Read the model definition and answer for the solid it produces. Units are mm, in the model's axes. Give positions to 0.01 mm unless a question says otherwise; leave off trailing zeros. Order: outer loops, then holes, each group sorted by start corner. A loop starts at its lowest first (then second) coordinate and runs counter-clockwise, first axis right, second up. Notation, with made-up numbers: (-18.5, -2.75) - (38.5, -2.75) arc R14 cw to (38.5, 5.25) - close; hole circle Ø9 at (-36.75, 85.5). An arc over 180 degrees is marked (long way). Write item = value, one per line.
```python
from build123d import *

# Parameters (mm, degrees)
F0_W     = 1250
F0_H     = 450
F1_DEPTH = 19
F3_DEPTH = 19
F5_DEPTH = 19
F7_D     = 10
F7_DEPTH = 13
F7_TIP   = 3.0043030951


with BuildPart() as f1:
    # F0 (on Top) → F1 (new body)
    with BuildSketch(Plane.XY):
        Rectangle(F0_W, F0_H)
    extrude(amount=F1_DEPTH)

    # F2 (on face) → F3 (cut, through all)
    with BuildSketch(Plane.XY.offset(19)):
        with BuildLine():
            Line((-190, 225), (-370, 225))
            Line((-370, 225), (-329.0003629481, 23.0519132014))
            ThreePointArc((-329.0003629481, 23.0519132014), (-280, -17), (-230.9996370519, 23.0519132014))
            Line((-230.9996370519, 23.0519132014), (-190, 225))
        make_face()
    extrude(amount=-F3_DEPTH, mode=Mode.SUBTRACT)

    # F4 (on face) → F5 (cut, through all)
    with BuildSketch(Plane.XY.offset(19)):
        with BuildLine():
            Line((385, 225), (205, 225))
            Line((205, 225), (240.8919167139, 28.1351470815))
            ThreePointArc((240.8919167139, 28.1351470815), (295, -17), (349.1080832861, 28.1351470815))
            Line((349.1080832861, 28.1351470815), (385, 225))
        make_face()
    extrude(amount=-F5_DEPTH, mode=Mode.SUBTRACT)

    # F7
    with Locations(Plane(origin=(0, 0, 0), x_dir=(1, 0, 0), z_dir=(0, 0, -1))):
        with Locations((-613, 150), (-175, 150), (175, 150), (613, 150), (-613, -150), (-175, -150), (175, -150), (613, -150)):
            Hole(F7_D / 2, depth=F7_DEPTH)
            with Locations((0, 0, -(F7_DEPTH + F7_TIP / 2))):  # 118° drill point
                Cone(0, F7_D / 2, F7_TIP, mode=Mode.SUBTRACT)


solid = f1.part
```
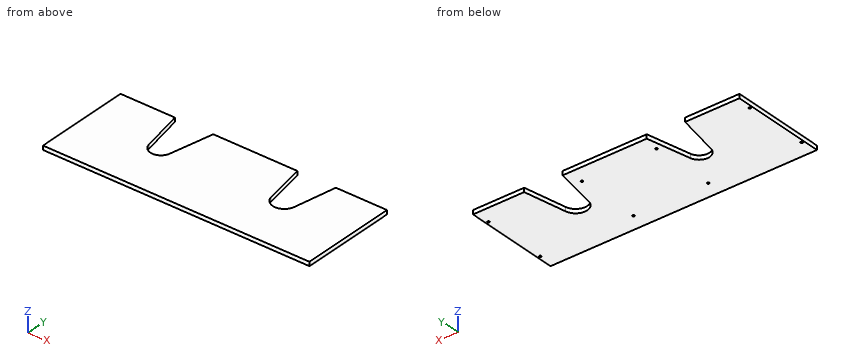
1. Section A-A (z = 3.25) is taken. Count the separate pieces of the cut face and the enclosed holes in it, and give its area (3 significant figures).
Recorded:
separate_pieces = 1
enclosed_holes = 8
area = 499,000 mm^2
2. Section B-B (y = 73) is taken. Determine the outline of the cut face in (x, z).
Recorded:
outline = (-625, 0) - (-339.14, 0) - (-339.14, 19) - (-625, 19) - close; (-220.86, 0) - (232.71, 0) - (232.71, 19) - (-220.86, 19) - close; (357.29, 0) - (625, 0) - (625, 19) - (357.29, 19) - close
3. Straight lines are drawn through the part: L1, parallel to X at y = -150, z = 6; L2, parallel to Y at x = 175, z = 6.25; L3, parallel to X at y = 196, z = 11. For each, find the intervals that lie inside material, in ascending order. Write a range as [from, to].
Recorded:
L1 = [-625, -618], [-608, -180], [-170, 170], [180, 608], [618, 625]
L2 = [-225, -155], [-145, 145], [155, 225]
L3 = [-625, -364.11], [-195.89, 210.29], [379.71, 625]
4. Section C-C (x = 256) is taken. Determine the outline of the cut face in (y, z).
Recorded:
outline = (-225, 0) - (-0.78, 0) - (-0.78, 19) - (-225, 19) - close
5. Flat-ended cylindrical pins translate along their axes: pin 1 (8 mm diameter, centred on x = 613, y = 150, fed in from -Z); pin 2 (3 mm diameter, centred on x = 294.5, z = 13.5, fed in from +Y). Find the tip coordinate at first contact, or state that the pin passes through.
Recorded:
pin_1 = 13.6
pin_2 = -16.96
